Input: part model. Units: mm. Frame: model coordinates. A direction names the side the tool comes from. Coordinates: 2 decimals unless noted, no trailing zeros. Loops run counter-clockwise (first coordinate to the right, second up) from the corner with the lowest first, then second, coordinate; pieces in that order, holes last.
(1) Mould query, pull axis Z, two halves, no side actions, for faces 4 (the face through (-1, -18.999, 15)), 5 (the face through (22.46, -0.24, 1.53)), 6 (the face through (20.64, 17.31, 12.81)), 7 (the face through (-24.014, -18.235, 12.842)). Classes: released by +Z, released by -Z, zero draft, split by the parting line, or undercut.
(2) Set-up query: faces 1 (the face through (-3.9, -20.09, 1.53)), 2 (the face through (-2.65, 17.345, 3.304)), 3 (the face through (-22.198, -2, 24)). Return all of +Z, -Z, +X, -X, +Y, -Y with unobstructed straight access to the full face (end or side cutting, diameter ignored); none if empty.
(3) Section A-A, the plane y = -8. Return loops of the section in (x, z), then the cut area to 3 significant figures.
(4) Contact query for flat-ended pins moving along their axis: P1, Ø2, axis at y = 2.5, z = 24, coming from the +X side; P2, Ø3, axis at y = 4, z = 23.5, coming from the -X side; P3, Ø16, axis at x = 6.5, y = 0, coming from the +Z side. Output: stop coordinate, or through.
(5) Section D-D, the plane y = 16.5. Return loops of the section in (x, z), then the cut area to 3 significant figures.
(6) Line query: L1, parallel to X at y = 9, z = 8.75; L2, parallel to Y at x = 13, z = 11.5; L3, parallel to Z at x = -18, y = -7.5. Output: solid intervals per line, ascending.
(7) Section C-C, the plane x = 18. Return loops of the section in (y, z), then the cut area to 3 significant figures.
(8) Section B-B, the plane z = 15. Return loops of the section in (x, y).
```python
from build123d import *

# Parameters (mm, degrees)
F0_W     = 51.1847995222
F0_H     = 42.1479381621
F1_DEPTH = 25.4
F2_R     = 5.08
F3_T     = -2.54


# Not quite as in the source:
# - a shell that OpenCascade refuses in one call is made with other operations: the cavity is built on its own and cut out


with BuildPart() as f1:
    # F0 (on Top) → F1 (new body)
    with BuildSketch(Plane.XY):
        with Locations((-1.6854219139, -0.4646256566)):
            Rectangle(F0_W, F0_H)
    extrude(amount=F1_DEPTH)

    # F2
    f2_edges = [f1.edges().sort_by_distance(p)[0] for p in [
        (-1.685422, 20.609343, 25.4),
        (-27.277822, -0.464626, 25.4),
        (23.906978, -0.464626, 25.4),
        (23.906978, -0.464626, 0),
        (23.906978, 20.609343, 12.7),
        (23.906978, -21.538595, 12.7),
        (-27.277822, 20.609343, 12.7),
        (-1.685422, -21.538595, 0),
        (-27.277822, -21.538595, 12.7),
        (-1.685422, 20.609343, 0),
    ]]
    fillet(f2_edges, radius=F2_R)

    # F3: a shell. OpenCascade refuses it in one call, so the cavity is built on its own and cut out:
    # the body offset inwards by the wall thickness, plus a prism from it out through each open face.
    f3_core = offset(f1.part, amount=F3_T, mode=Mode.PRIVATE)
    f3_exits = [f3_core.faces().sort_by_distance(p)[0] for p in [
        (-1.685422, -1.734626, 22.86),
    ]]
    add(f3_core, mode=Mode.SUBTRACT)
    extrude(f3_exits, amount=-F3_T, mode=Mode.SUBTRACT)


solid = f1.part
```
Report:
1. face 4: zero draft
1. face 5: released by -Z
1. face 6: undercut
1. face 7: undercut
2. face 1: -Z, +X, -X, -Y
2. face 2: none
2. face 3: +Z
3. outline: (-27.28, 0) - (18.83, 0) arc R5.08 ccw to (23.91, 5.08) - (23.91, 20.32) arc R5.08 ccw to (18.83, 25.4) - (18.83, 22.86) arc R2.54 cw to (21.37, 20.32) - (21.37, 5.08) arc R2.54 cw to (18.83, 2.54) - (-24.74, 2.54) - (-24.74, 20.32) arc R2.54 cw to (-22.2, 22.86) - (-22.2, 25.4) arc R5.08 ccw to (-27.28, 20.32) - close
3. area: 247 mm2
4. P1: stops at x = 23.14
4. P2: stops at x = -26.99
4. P3: stops at z = 2.54
5. outline: (-27.18, 0.09) - (18.83, 0.09) arc R4.99 ccw to (23.81, 5.08) - (23.81, 20.32) arc R4.99 ccw to (18.83, 25.31) - (-22.2, 25.31) arc R4.99 ccw to (-27.18, 20.32) - close; hole (-24.55, 2.73) - (18.83, 2.73) arc R2.35 ccw to (21.17, 5.08) - (21.17, 20.32) arc R2.35 ccw to (18.83, 22.67) - (-22.2, 22.67) arc R2.35 ccw to (-24.55, 20.32) - close
5. area: 362 mm2
6. L1: x = -27.28 to -24.74, 21.37 to 23.91
6. L2: y = -21.54 to -19, 18.07 to 20.61
6. L3: z = 0 to 2.54
7. outline: (-21.54, 5.08) arc R5.08 ccw to (-16.46, 0) - (15.53, 0) arc R5.08 ccw to (20.61, 5.08) - (20.61, 20.32) arc R5.08 ccw to (15.53, 25.4) - (15.53, 22.86) arc R2.54 cw to (18.07, 20.32) - (18.07, 5.08) arc R2.54 cw to (15.53, 2.54) - (-16.46, 2.54) arc R2.54 cw to (-19, 5.08) - (-19, 25.4) - (-21.54, 25.4) - close
7. area: 217 mm2
8. outline: (-27.28, -16.46) arc R5.08 ccw to (-22.2, -21.54) - (18.83, -21.54) arc R5.08 ccw to (23.91, -16.46) - (23.91, 15.53) arc R5.08 ccw to (18.83, 20.61) - (-22.2, 20.61) arc R5.08 ccw to (-27.28, 15.53) - close; hole (-24.74, -16.46) arc R2.54 ccw to (-22.2, -19) - (18.83, -19) arc R2.54 ccw to (21.37, -16.46) - (21.37, 15.53) arc R2.54 ccw to (18.83, 18.07) - (-22.2, 18.07) arc R2.54 ccw to (-24.74, 15.53) - close
